```python
from build123d import *

# Parameters (mm, degrees)
SKETCH1_W           = 25.4
SKETCH1_H           = 25.4
SKETCH1_W_2         = 19.05
SKETCH1_H_2         = 19.05
BOSS_EXTRUDE1_DEPTH = 101.6
SKETCH2_W           = 25.4
SKETCH2_H           = 26.296014983
CUT_EXTRUDE1_DEPTH  = 101.161834767
SKETCH5_W           = 25.4
SKETCH5_H           = 29.329393675
CUT_EXTRUDE2_DEPTH  = 90.577773471


with BuildPart() as part:
    # Sketch1 → Boss-Extrude1 (new body)
    with BuildSketch(Plane.XY):
        Rectangle(SKETCH1_W, SKETCH1_H)
        Rectangle(SKETCH1_W_2, SKETCH1_H_2, mode=Mode.SUBTRACT)
    extrude(amount=BOSS_EXTRUDE1_DEPTH)

    # Sketch2 → Cut-Extrude1 (cut, through all)
    with BuildSketch(Plane(origin=(-0.850738686, 0, 3.175), x_dir=(0, -1, 0), z_dir=(0.25881904510252135, 0, -0.9659258262890681))):
        with Locations((0, -0.880749498)):
            Rectangle(SKETCH2_W, SKETCH2_H)
    extrude(amount=CUT_EXTRUDE1_DEPTH, mode=Mode.SUBTRACT)

    # Sketch5 → Cut-Extrude2 (cut, through all)
    with BuildSketch(Plane(origin=(40.819090512, 0, 70.700738686), x_dir=(0, -1, 0), z_dir=(0.4999999999999889, 0, 0.866025403784445))):
        with Locations((0, -47.13382579)):
            Rectangle(SKETCH5_W, SKETCH5_H)
    extrude(amount=CUT_EXTRUDE2_DEPTH, mode=Mode.SUBTRACT)


solid = part.part
```
For this review, take the finished solid that the model builds, in its own axes (mm). A direction names the side the tool comes from. Coordinates: 2 decimals unless noted, no trailing zeros. Order: outer loops, then holes, each group sorted by start corner. A loop starts at its lowest first (then second) coordinate and runs counter-clockwise, first axis right, second up. Notation, with made-up numbers: (67.5, 60) -> (97.5, 60) arc R18 ccw to (97.5, 90) -> close; hole circle Ø4 at (9, 66). An arc over 180 degrees is marked (long way). Use CSV: the item, a comma, the result in double quotes. Start each with the question number.
Item 1: Wall thickness on probe 1 along Y at (x, z) = (3.5, 80.5) (3 decimals); probe 2 along X at (y, z) = (-7, 95.5) (3 decimals): over which ranges is each line inside the solid? List them lowest first.
Item 2: We need section A-A, the plane z = 13. Give the boundary of the cut face in (x, y) (3 decimals).
Item 3: Draft analysis for pull direction X (two halves, no side actions). For faces 1 (the face through (-9.525, 0, 50)), 2 (the face through (0.178, -11.111, 94.165)), 3 (the face through (0, -12.7, 50)), state which applies: pulls with the +X half, pulls with the -X half, needs draft (parallel to the pull), parting line crosses it, or undercut.
Item 4: We need section D-D, the plane z = 93.5. Give the boundary of the cut face in (x, y) (3 decimals).
Item 5: We need section C-C, the plane x = 7.75. Give the boundary of the cut face in (y, z) (3 decimals), then the cut area to 3 significant figures.
Item 6: For faces 4 (the face through (9.525, 0, 47)), 5 (the face through (0, 12.7, 50)), list the 3-axis set-ups (+Z, -Z, +X, -X, +Y, -Y) from which the entire face can be reached by the end or side of a thin tool; tool diameter is ignored.
Item 7: We need section B-B, the plane y = -8. Give the boundary of the cut face in (x, z) (3 decimals), then the cut area to 3 significant figures.
Item 8: Insertion check: pin 1 (12 mm diameter, centred on x = -5.5, y = 9.5, fed in from +Z); pin 2 (4 mm diameter, centred on x = 8, y = -4, fed in from +Z); pin 3 (3 mm diameter, centred on x = -8.5, y = -1.5, fed in from -Z). Each pin has a flat end and moves straight along its axis. Give the tip position at first contact, or say it passes through.
Derived:
1,probe 1,"y = -12.7 to -9.525, 9.525 to 12.7"
1,probe 2,"x = -12.7 to -9.525"
2,outline,"(-12.7, -12.7) -> (12.7, -12.7) -> (12.7, 12.7) -> (-12.7, 12.7) -> close; hole (-9.525, -9.525) -> (9.525, -9.525) -> (9.525, 9.525) -> (-9.525, 9.525) -> close"
3,face 1,"undercut"
3,face 2,"pulls with the +X half"
3,face 3,"needs draft"
4,outline,"(-12.7, -12.7) -> (1.33, -12.7) -> (1.33, -9.525) -> (-9.525, -9.525) -> (-9.525, 9.525) -> (1.33, 9.525) -> (1.33, 12.7) -> (-12.7, 12.7) -> close"
5,outline,"(-12.7, 5.48) -> (-9.525, 5.48) -> (-9.525, 89.793) -> (-12.7, 89.793) -> close; (9.525, 5.48) -> (12.7, 5.48) -> (12.7, 89.793) -> (9.525, 89.793) -> close"
5,area,"535 mm^2"
6,face 4,"+Z, -Z"
6,face 5,"+Z, -Z, +X, -X, +Y"
7,outline,"(-12.7, 0) -> (-9.525, 0.851) -> (-9.525, 99.767) -> (-12.7, 101.6) -> close; (9.525, 5.955) -> (12.7, 6.806) -> (12.7, 86.935) -> (9.525, 88.768) -> close"
7,area,"577 mm^2"
8,pin 1,"stops at z = 100.91"
8,pin 2,"stops at z = 88.77"
8,pin 3,"stops at z = 0.72"
